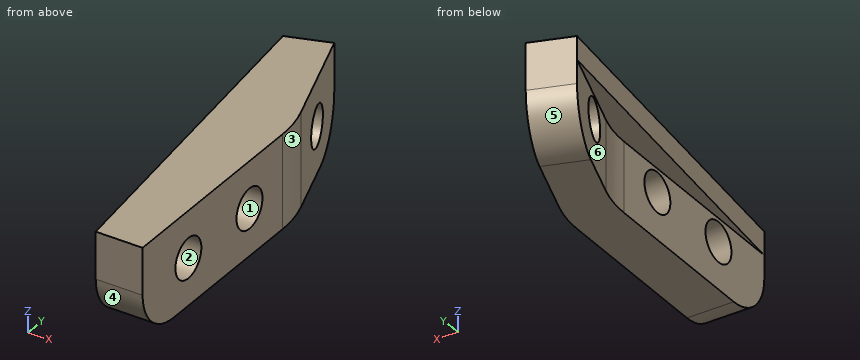
```python
from build123d import *

# Parameters (mm, degrees)
F0_W     = 2
F0_H     = 10
F1_DEPTH = 4
F3_DEPTH = 1
F4_R     = 0.85
F5_DEPTH = 25
F6_R     = 0.85
F7_DEPTH = 25
F8_R     = 5
F9_R     = 5
F10_R    = 2


with BuildPart() as f1:
    # F0 (on Top) → F1 (new body)
    with BuildSketch(Plane.XY):
        Polygon((-14.343983, 1.605531), (-12.731962, -3.12748), (-10.731962, -3.12748), (-12.551871, 2.215907), align=None)
        with Locations((-11.731962, -8.12748)):
            Rectangle(F0_W, F0_H)
    extrude(amount=F1_DEPTH)

    # F2 (on face) → F3 (join)
    with BuildSketch(Plane.XY.offset(4)):
        Polygon((-12.731962, -3.12748), (-14.343983, 1.605531), (-12.731962, -13.12748), align=None)
    extrude(amount=-F3_DEPTH)

    # F4 (on face) → F5 (cut)
    with BuildSketch(Plane(origin=(-12.363017, -4.210731, 0), x_dir=(0.322404, -0.946602, 0), z_dir=(-0.946602, -0.322404, 0))):
        with Locations((-3.644357, 2)):
            Circle(F4_R)
    extrude(amount=-F5_DEPTH, mode=Mode.SUBTRACT)

    # F6 (on face) → F7 (cut)
    with BuildSketch(Plane(origin=(-12.731962, 0, 0), x_dir=(0, -1, 0), z_dir=(-1, 0, 0))):
        with Locations((6.12748, 2)):
            Circle(F6_R)
        with Locations((10.12748, 2)):
            Circle(F6_R)
    extrude(amount=-F7_DEPTH, mode=Mode.SUBTRACT)

    # F8
    f8_edges = [f1.edges().sort_by_distance(p)[0] for p in [
        (-12.731962, -3.12748, 1.5),
    ]]
    fillet(f8_edges, radius=F8_R)

    # F9
    f9_edges = [f1.edges().sort_by_distance(p)[0] for p in [
        (-10.731962, -3.12748, 2),
    ]]
    fillet(f9_edges, radius=F9_R)

    # F10
    f10_edges = [f1.edges().sort_by_distance(p)[0] for p in [
        (-11.731962, -13.12748, 0),
        (-13.447927, 1.910719, 0),
    ]]
    fillet(f10_edges, radius=F10_R)


solid = f1.part
```
Geometry check sheet. Reference: the model listing, model coordinates, mm. Face numbers are marked on the shaded views. A direction names the side the tool comes from. Coordinates: 2 decimals unless noted, no trailing zeros. Order: outer loops, then holes, each group sorted by start corner. A loop starts at its lowest first (then second) coordinate and runs counter-clockwise, first axis right, second up. Notation, with made-up numbers: (3, 89) - (60, 89) arc R26 cw to (60, 118) - close; hole circle Ø8 at (10.25, 10). An arc over 180 degrees is marked (long way). Answer in a Markdown table with one row per item. Add a question column.
1. Section check A-A (y = -11.5). Enter the section's corners in (x, z) (3 decimals), plus the area to 3 significant figures.
2. Access from +Z, -Z, +X, -X, +Y, -Y to the whole of each face (thin tool, end or side, straight path). Record for the marked faces 5 and 6.
3. Draft check along Z on the marked faces 1, 2, 3 and 4. Enter one of: +Z half, -Z half, draft (parallel to the pull), parting line (faces both ways), or undercut.
4. Section check C-C (x = -11.75). Give the number of separate pieces and of enclosed holes in the cut face, plus the area to 3 significant figures.
5. Material ranges on L1, parallel to Y at x = -11.7, z = 1.45; L2, parallel to X at y = -5.5, z = 1.3; L3, parallel to Y at x = -12.6, z = 1.6, recorded low to high. Write a range as [from, to].
6. Gauge pin test, flat ends, axial feed: pin 1 Ø0.8 at (x, y) = (-13.5, -7) entering from -Z; pin 2 Ø1.5 at (x, z) = (-13.5, 0.5) entering from +Y; pin 3 Ø1 at (y, z) = (-6.13, 2) entering from +X. Record the tip position at first contact, or that the pin passes through.
7. Section check B-B (z = 0.65). Enter the section's corners in (x, y), plus the area to 3 significant figures.
8. Section check D-D (y = -7.5). Enter the section's corners in (x, z), plus the area to 3 significant figures.
Data:
| question | item | result |
|---|---|---|
| 1 | outline | (-12.91, 3) - (-12.732, 3) - (-12.732, 0.035) - (-10.732, 0.035) - (-10.732, 4) - (-12.91, 4) - close |
| 1 | area | 8.11 mm² |
| 2 | face 5 | -Z, -X, +Y |
| 2 | face 6 | -Z, -X, -Y |
| 3 | face 1 | undercut |
| 3 | face 2 | undercut |
| 3 | face 3 | draft |
| 3 | face 4 | -Z half |
| 4 | separate pieces | 1 |
| 4 | enclosed holes | 2 |
| 4 | area | 45.3 mm² |
| 5 | L1 | y = [-13.05, -10.78], [-9.48, -6.78], [-5.48, -0.82] |
| 5 | L2 | x = [-12.73, -10.73] |
| 5 | L3 | y = [-13.09, -10.88], [-9.38, -6.88], [-5.38, -1.23], [0.35, 2.16] |
| 6 | pin 1 | stops at z = 3 |
| 6 | pin 2 | stops at y = 1.82 |
| 6 | pin 3 | passes through |
| 7 | outline | (-14.17, 1.11) - (-13, -2.34) arc R5 cw to (-12.73, -3.96) - (-12.73, -12.6) - (-10.73, -12.6) - (-10.73, -3.96) arc R5 ccw to (-11, -2.34) - (-12.38, 1.72) - close |
| 7 | area | 28.0 mm² |
| 8 | outline | (-13.35, 3) - (-12.73, 3) - (-12.73, 0) - (-10.73, 0) - (-10.73, 4) - (-13.35, 4) - close |
| 8 | area | 8.62 mm² |
